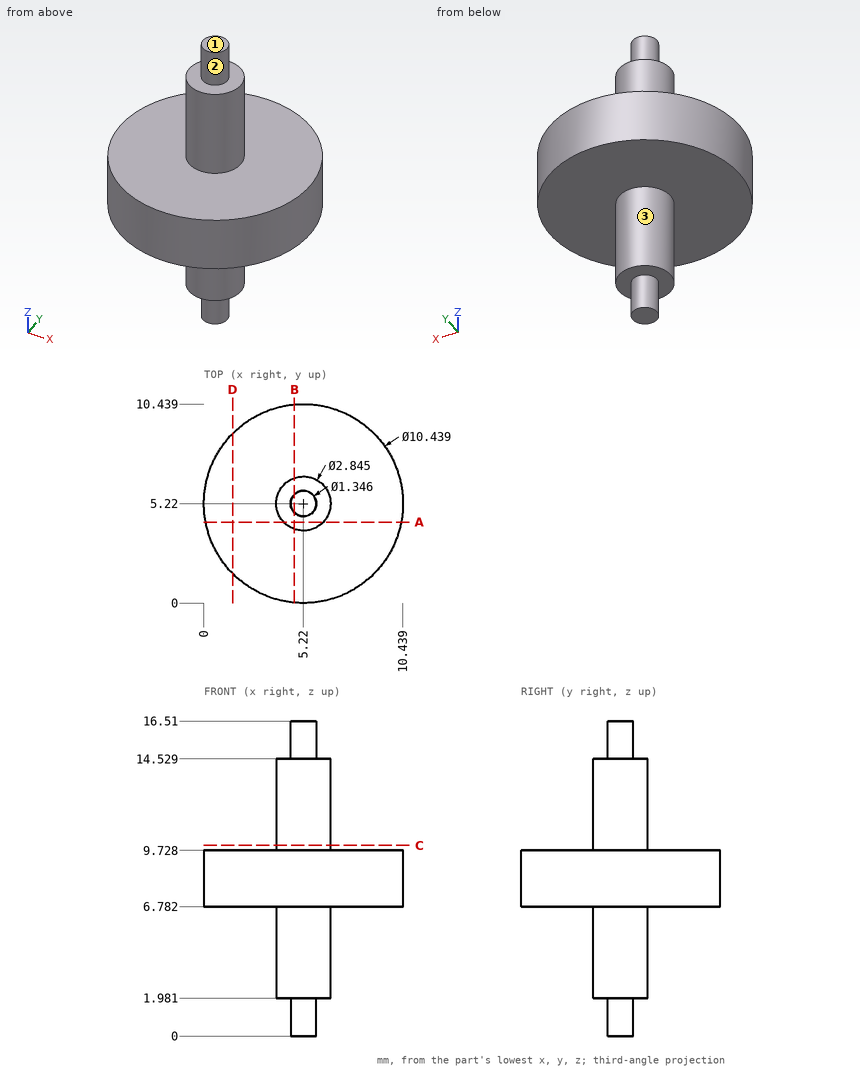
Design review of the part shown in the three views and the two pictorial views. Dimensions are in mm from the part's minimum x, y and z. A direction names the side the tool comes from. Coordinates: 2 decimals unless noted, no trailing zeros. Write each loop counter-clockwise with the first axis right and the second up, starting at its lowest first coordinate (ties: lowest second). Pieces come first, ordered by that corner, then holes.
(1) Add section A-A on y = 4.25. Give the boundary of the cut face in (x, z), then the cut area to 3 significant figures.
(2) Wall thickness on probe 1 along X at (y, z) = (5.25, 14.75); probe 2 along Y at (x, z) = (5.25, 6.75); probe 3 along Z at (x, y) = (6, 2.75): over which ranges is each line inside the solid? List them lowest first.
(3) For pin 1 Ø4 at (x, z) = (7, 5) entering from -Y; pin 2 Ø3 at (x, z) = (9, 4.5) entering from -Y; pin 3 Ø3 at (x, y) = (6.5, 6.5) entering from -Z; pin 4 Ø3 at (x, z) = (7.5, 11.5) entering from -Y, all flat-tipped, find the tip position at first contact; note any pin that passes through.
(4) Tool access review of the marked faces 1, 2 and 3: name each direction out of +Z, -Z, +X, -X, +Y, -Y from which nothing blocks a thin tool from reaching the whole face with its end or side.
(5) Add section C-C on z = 10. Give the boundary of the cut face in (x, y) (1 decimal).
(6) Add section B-B on x = 4.75. Give the boundary of the cut face in (y, z).
(7) Add section D-D on x = 1.5. Give the boundary of the cut face in (y, z), then the cut area to 3 significant figures.
Answer sheet:
1. outline: (0.09, 6.78) - (4.18, 6.78) - (4.18, 1.98) - (6.26, 1.98) - (6.26, 6.78) - (10.35, 6.78) - (10.35, 9.73) - (6.26, 9.73) - (6.26, 14.53) - (4.18, 14.53) - (4.18, 9.73) - (0.09, 9.73) - close
1. area: 50.2 mm2
2. probe 1: x = 4.55 to 5.89
2. probe 2: y = 3.8 to 6.64
2. probe 3: z = 6.78 to 9.73
3. pin 1: stops at y = 0.07
3. pin 2: passes through
3. pin 3: stops at z = 0
3. pin 4: stops at y = 4.03
4. face 1: +Z, +X, -X, +Y, -Y
4. face 2: +Z
4. face 3: -Z
5. outline: circle Ø2.8 at (5.2, 5.2)
6. outline: (0.02, 6.78) - (3.88, 6.78) - (3.88, 1.98) - (4.74, 1.98) - (4.74, 0) - (5.7, 0) - (5.7, 1.98) - (6.56, 1.98) - (6.56, 6.78) - (10.42, 6.78) - (10.42, 9.73) - (6.56, 9.73) - (6.56, 14.53) - (5.7, 14.53) - (5.7, 16.51) - (4.74, 16.51) - (4.74, 14.53) - (3.88, 14.53) - (3.88, 9.73) - (0.02, 9.73) - close
7. outline: (1.56, 6.78) - (8.88, 6.78) - (8.88, 9.73) - (1.56, 9.73) - close
7. area: 21.6 mm2
